Geometry: final body of the model. Coordinates: model frame, mm. Give positions to 0.01 mm unless a question says otherwise; leave off trailing zeros. Write each loop counter-clockwise with the first axis right and the second up, starting at its lowest first coordinate (ties: lowest second). Pieces come first, ordered by that corner, then holes. Notation, with made-up numbers: M -32,31 L -14,31 A14 cw -14,55 Z; hole C 62.5,52.5 d11. An arc over 180 degrees is marked long. Use a Markdown table: item, result. Add a question column.
(1) Cut plane B-B (z = -36.5). Output: boundary loops of the cut face in (x, y), plus the area to 3 significant figures.
(2) Material intervals for L1, parallel to Z at x = 253, y = 0.5; L2, parallel to X at y = 2.5, z = -125.5; L3, parallel to X at y = 5, z = -76.2, sorted ascending.
(3) Cut plane D-D (x = 283). Output: boundary loops of the cut face in (y, z).
(4) Cut plane C-C (x = 242.5). Output: boundary loops of the cut face in (y, z), plus the area to 3 significant figures.
(5) Cut plane A-A (y = 2.5). Output: boundary loops of the cut face in (x, z), plus the area to 3 significant figures.
(6) Pin query (flat end, axial travel): pin 1 Ø12 at (x, z) = (123.5, -60.5) entering from -Y. Return the tip coordinate at first contact, or that it passes through.
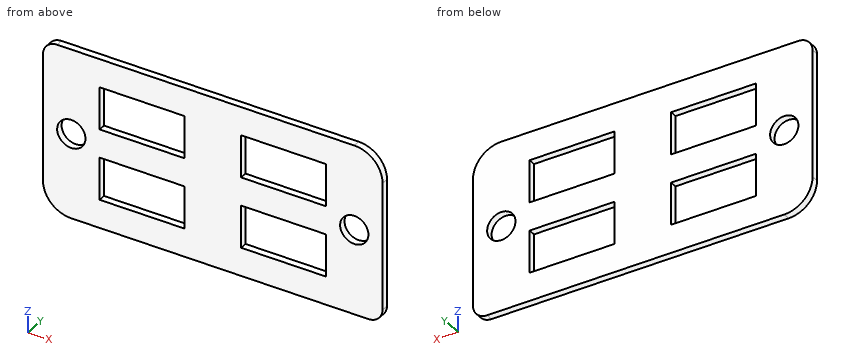
```python
from build123d import *

# Parameters (mm, degrees)
SKETCH1_W           = 304.8
SKETCH1_H           = 152.4
SKETCH1_R           = 12.7
SKETCH1_W_2         = 76.2
SKETCH1_H_2         = 38.1
BOSS_EXTRUDE1_DEPTH = 6.35
FILLET2_R           = 25.4
FILLET3_R           = 12.7


with BuildPart() as part:
    # Sketch1 → Boss-Extrude1 (new body)
    with BuildSketch(Plane(origin=(0, 0, 0), x_dir=(1, 0, 0), z_dir=(0, 1, 0))):
        with Locations((152.4, 76.2)):
            Rectangle(SKETCH1_W, SKETCH1_H)
        with Locations(Location((25.4, 76.2, 0), (0, 0, 270))):
            Circle(SKETCH1_R, mode=Mode.SUBTRACT)
        with Locations(Location((279.4, 76.2, 0), (0, 0, 270))):
            Circle(SKETCH1_R, mode=Mode.SUBTRACT)
        with Locations((88.9, 107.95)):
            Rectangle(SKETCH1_W_2, SKETCH1_H_2, mode=Mode.SUBTRACT)
        with Locations((88.9, 44.45)):
            Rectangle(SKETCH1_W_2, SKETCH1_H_2, mode=Mode.SUBTRACT)
        with Locations((215.9, 107.95)):
            Rectangle(SKETCH1_W_2, SKETCH1_H_2, mode=Mode.SUBTRACT)
        with Locations((215.9, 44.45)):
            Rectangle(SKETCH1_W_2, SKETCH1_H_2, mode=Mode.SUBTRACT)
    extrude(amount=BOSS_EXTRUDE1_DEPTH)

    # Fillet2
    fillet2_edges = [part.edges().sort_by_distance(p)[0] for p in [
        (0, 3.175, -152.4),
        (304.8, 3.175, 0),
    ]]
    fillet(fillet2_edges, radius=FILLET2_R)

    # Fillet3
    fillet3_edges = [part.edges().sort_by_distance(p)[0] for p in [
        (304.8, 3.175, -152.4),
        (0, 3.175, 0),
    ]]
    fillet(fillet3_edges, radius=FILLET3_R)


solid = part.part
```
Answer list:
| question | item | result |
|---|---|---|
| 1 | outline | M 0,0 L 50.8,0 L 50.8,6.35 L 0,6.35 Z; M 127,0 L 177.8,0 L 177.8,6.35 L 127,6.35 Z; M 254,0 L 304.8,0 L 304.8,6.35 L 254,6.35 Z |
| 1 | area | 968 mm² |
| 2 | L1 | -152.4 to -127, -88.9 to -63.5, -25.4 to 0 |
| 2 | L2 | 0 to 50.8, 127 to 177.8, 254 to 304.8 |
| 2 | L3 | 0 to 12.7, 38.1 to 266.7, 292.1 to 304.8 |
| 3 | outline | M 0,-152.4 L 6.35,-152.4 L 6.35,-88.38 L 0,-88.38 Z; M 0,-64.02 L 6.35,-64.02 L 6.35,-0.26 L 0,-0.26 Z |
| 4 | outline | M 0,-152.4 L 6.35,-152.4 L 6.35,-127 L 0,-127 Z; M 0,-88.9 L 6.35,-88.9 L 6.35,-63.5 L 0,-63.5 Z; M 0,-25.4 L 6.35,-25.4 L 6.35,0 L 0,0 Z |
| 4 | area | 484 mm² |
| 5 | outline | M 0,-127 A25.4 ccw 25.4,-152.4 L 292.1,-152.4 A12.7 ccw 304.8,-139.7 L 304.8,-25.4 A25.4 ccw 279.4,0 L 12.7,0 A12.7 ccw 0,-12.7 Z; hole C 25.4,-76.2 d25.4; hole M 50.8,-127 L 127,-127 L 127,-88.9 L 50.8,-88.9 Z; hole M 50.8,-63.5 L 127,-63.5 L 127,-25.4 L 50.8,-25.4 Z; hole M 177.8,-127 L 254,-127 L 254,-88.9 L 177.8,-88.9 Z; hole M 177.8,-63.5 L 254,-63.5 L 254,-25.4 L 177.8,-25.4 Z; hole C 279.4,-76.2 d25.4 |
| 5 | area | 33,500 mm² |
| 6 | pin 1 | y = 0 |
